Part model, mm, in its own coordinate system. Face numbers are marked on the shaded views. A direction names the side the tool comes from. Give positions to 0.01 mm unless a question says otherwise; leave off trailing zeros. Write each loop counter-clockwise with the first axis right and the second up, starting at its lowest first coordinate (ties: lowest second). Pieces come first, ordered by that corner, then holes.
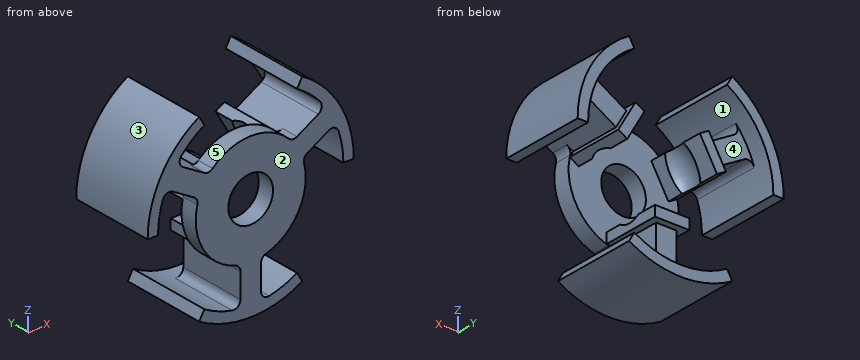
from build123d import *

# Parameters (mm, degrees)
SKETCH_1_R               = 16
SKETCH_1_R_2             = 6.5
EXTRUDE_1_DEPTH          = 5
SKETCH_2_W               = 10
SKETCH_2_H               = 3
EXTRUDE_2_DEPTH          = 22
EXTRUDE_3_DEPTH          = 25
EXTRUDE_4_DEPTH          = 20
FILLET_1_R               = 2
FILLET_2_R               = 2
FILLET_3_R               = 2
FILLET_4_R               = 2
PATTERN_CIRCULAR_4_COUNT = 3
PATTERN_CIRCULAR_5_COUNT = 3
FILLET_5_R               = 2


with BuildPart() as part:
    # Sketch 1 → Extrude 1 (new body)
    with BuildSketch(Plane(origin=(0, 0, 0), x_dir=(1, 0, 0), z_dir=(0, 1, 0))):
        with Locations(Location((0, 0, 0), (0, 0, 270))):
            Circle(SKETCH_1_R)
        with Locations(Location((0, 0, 0), (0, 0, 270))):
            Circle(SKETCH_1_R_2, mode=Mode.SUBTRACT)
    extrude(amount=EXTRUDE_1_DEPTH)

    # Sketch 2 → Extrude 2 (add)
    with BuildSketch(Plane(origin=(0, 0, 0), x_dir=(1, 0, 0), z_dir=(0, 1, 0))):
        with Locations((-1.78e-15, 13.698684153570664)):
            Rectangle(SKETCH_2_W, SKETCH_2_H)
    extrude_2 = extrude(amount=EXTRUDE_2_DEPTH)



with BuildPart() as body_2:
    # Sketch 3 → Extrude 3 (new body)
    with BuildSketch(Plane(origin=(0, 0, 0), x_dir=(1, 0, 0), z_dir=(0, 1, 0))):
        with BuildLine():
            Line((-15.000000000000039, 25.98076211353314), (-13.484105265359647, 23.355155414209925))
            ThreePointArc((-13.484105265359647, 23.355155414209925), (1.65e-15, 26.968210530719293), (13.484105265359647, 23.355155414209925))
            Line((13.484105265359647, 23.355155414209925), (15.000000000000039, 25.98076211353314))
            ThreePointArc((15.000000000000039, 25.98076211353314), (1.84e-15, 30), (-15.000000000000039, 25.98076211353314))
        make_face()
    extrude_3 = extrude(amount=EXTRUDE_3_DEPTH)


with BuildPart() as part_1:
    add(part.part)

    add(body_2.part)  # Extrude 4 merges body 2
    # Sketch 4 → Extrude 4 (add)
    with BuildSketch(Plane(origin=(0, 0, 0), x_dir=(1, 0, 0), z_dir=(0, 1, 0))):
        Polygon((2.9999999999999964, 14.402885682574833), (-3.000000000000003, 14.402885682574832), (-3.0000000000000036, 27.990866329379006), (2.9999999999999964, 27.990866329379006), align=None)
    extrude_4 = extrude(amount=EXTRUDE_4_DEPTH)

    # Sketch 5 → Cut-Revolve 1 (revolve, cut)
    with BuildSketch(Plane(origin=(0, 0, 0), x_dir=(0, 0, -1), z_dir=(1, 0, 0))):
        with BuildLine():
            Line((12.198684153570664, 17.303207954702064), (8.4, 13))
            Line((8.4, 13), (12.198684153570664, 8.696792045297935))
            ThreePointArc((12.198684153570664, 8.696792045297935), (14.139999999999999, 13), (12.198684153570664, 17.303207954702064))
        make_face()
    cut_revolve_1 = revolve(axis=Axis((0, -2.5210076515236324, 0), (0, 1, 0)), mode=Mode.SUBTRACT)

    # Fillet 1
    fillet_1_edges = [part_1.edges().sort_by_distance(p)[0] for p in [
        (2.9999999999999964, 10, -26.80082795790456),
    ]]
    fillet(fillet_1_edges, radius=FILLET_1_R)

    # Fillet 2
    fillet_2_edges = [part_1.edges().sort_by_distance(p)[0] for p in [
        (-3.0000000000000036, 10, -26.80082795790456),
    ]]
    fillet(fillet_2_edges, radius=FILLET_2_R)

    # Fillet 3
    fillet_3_edges = [part_1.edges().sort_by_distance(p)[0] for p in [
        (-3.000000000000003, 2.5, -15.71623364550171),
    ]]
    fillet(fillet_3_edges, radius=FILLET_3_R)

    # Fillet 4
    fillet_4_edges = [part_1.edges().sort_by_distance(p)[0] for p in [
        (2.9999999999999964, 2.5, -15.716233645501712),
    ]]
    fillet(fillet_4_edges, radius=FILLET_4_R)

    # Pattern Circular 4: Extrude 2, Extrude 4, Cut-Revolve 1 ×3 about axis
    pattern_circular_4_axis = Axis((1.5e-16, 0, 7.6e-16), (0, 1, 0))
    add([extrude_2.rotate(pattern_circular_4_axis, i * 360 / PATTERN_CIRCULAR_4_COUNT) for i in range(1, PATTERN_CIRCULAR_4_COUNT)])
    add([extrude_4.rotate(pattern_circular_4_axis, i * 360 / PATTERN_CIRCULAR_4_COUNT) for i in range(1, PATTERN_CIRCULAR_4_COUNT)])
    add([cut_revolve_1.rotate(pattern_circular_4_axis, i * 360 / PATTERN_CIRCULAR_4_COUNT) for i in range(1, PATTERN_CIRCULAR_4_COUNT)], mode=Mode.SUBTRACT)

    # Pattern Circular 5: Extrude 3 ×3 about axis
    pattern_circular_5_axis = Axis((3.1e-16, 0, 6.1e-16), (0, 1, 0))
    for i in range(1, PATTERN_CIRCULAR_5_COUNT):
        add(extrude_3.rotate(pattern_circular_5_axis, i * 360 / PATTERN_CIRCULAR_5_COUNT))

    # Fillet 5
    fillet_5_edges = [part_1.edges().sort_by_distance(p)[0] for p in [
        (12.110657588816196, 2.5, 10.456193034104174),
        (15.110657588816197, 2.5, 5.260040611397544),
        (-15.110657588816201, 2.5, 5.260040611397544),
        (-12.110657588816197, 2.5, 10.456193034104171),
        (24.710197854001564, 10, 10.802337767598974),
        (21.71019785400156, 10, 15.998490190305604),
        (-21.71019785400157, 10, 15.998490190305594),
        (-24.71019785400157, 10, 10.802337767598964),
    ]]
    fillet(fillet_5_edges, radius=FILLET_5_R)


solid = part_1.part
1) Saw through at D-D (y = 6.25). State how many separate pieces and enclosed holes the cut face has, and give its area (3 significant figures).
Check result:
separate pieces: 3
enclosed holes: 0
area: 580 mm2
2) Drill centre lines: L1, parallel to X at y = 20.75, z = 4.5; L2, parallel to X at y = 7.5, z = 2; L3, parallel to X at y = 4.25, z = 21. Where is each one in solid material? Low to high.
Check result:
L1: x = -29.66 to -26.59, -14.95 to -11.49, 11.49 to 14.95, 26.59 to 29.66
L2: x = -29.93 to -26.89, -13.46 to -12.93, 12.93 to 13.46, 26.89 to 29.93
L3: x = -21.42 to -16.92, 16.92 to 21.42
3) 3-axis set-ups, long thin cutter, end or side, ignore diameter. For the marked faces 4 and 5: which of +Z, -Z, +X, -X, +Y, -Y reach the whole face in a straight line?
Check result:
face 4: +Y
face 5: +Z, +Y, -Y
4) Saw through at C-C (x = 24). Write the cut outline in (y, z), and give its area (3 significant figures).
Check result:
outline: (0, 9.88) - (20, 9.88) - (20, 12.3) - (25, 12.3) - (25, 18) - (0, 18) - close
area: 191 mm2
5) Saw through at A-A (x = 0). Write the cut outline in (y, z).
Check result:
outline: (0, -30) - (25, -30) - (25, -26.97) - (20, -26.97) - (20, -15.2) - (22, -15.2) - (22, -12.2) - (17.3, -12.2) arc R5.74 cw to (8.7, -12.2) - (5, -12.2) - (5, -6.5) - (0, -6.5) - close; (0, 6.5) - (5, 6.5) - (5, 16) - (0, 16) - close
6) Mould opens along X. For the marked faces 1, 2 and 3 say: +X half, -X half, draft (parallel to the pull), parting line (faces both ways), or undercut.
Check result:
face 1: undercut
face 2: draft
face 3: -X half
7) Flat gauge pins, fed straight in: P1, Ø3, axis at x = -1.5, y = 18, coming from the +Z side; P2, Ø2.5, axis at y = 15, z = -13, coming from the +X side; P3, Ø2.5, axis at x = 11.5, z = 9, coming from the +Y side; P4, Ø0.5, axis at x = -12.5, z = 11.5, coming from the +Y side. Where does each tip first touch, or does it go through?
Check result:
P1: stops at z = -12.2
P2: stops at x = 5
P3: stops at y = 22
P4: passes through
8) Saw through at B-B (z = -5). Write the cut outline in (x, y), and give its area (3 significant figures).
Check result:
outline: (-15.2, 0) - (-4.15, 0) - (-4.15, 5) - (-15.2, 5) - close; (4.15, 0) - (15.2, 0) - (15.2, 5) - (4.15, 5) - close
area: 110 mm2
